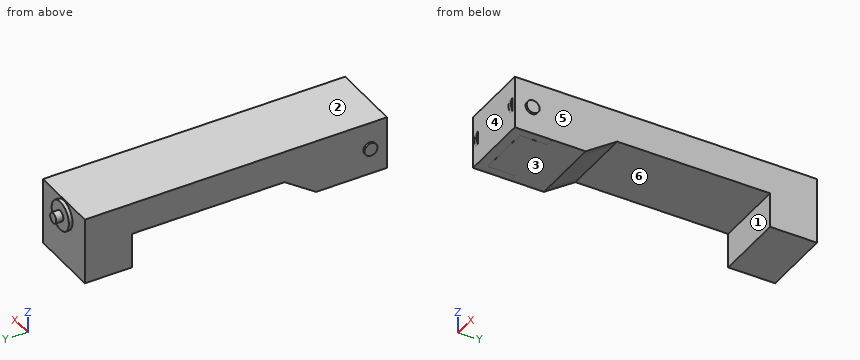
from build123d import *
from OCP.BRepFilletAPI import BRepFilletAPI_MakeChamfer

# Parameters (mm, degrees)
SKETCH1_W            = 41
SKETCH1_H            = 40.2
BOSS_EXTRUDE1_DEPTH  = 61.1
SKETCH2_R            = 14
BOSS_EXTRUDE2_DEPTH  = 3
SKETCH3_R            = 4.9
BOSS_EXTRUDE3_DEPTH  = 4.8
CHAMFER1_SIZE        = 7.5
CHAMFER1_SIZE2       = 5.1
MIRROR5_START        = -20.5
MIRROR5_DEPTH        = 41
BOSS_EXTRUDE4_DEPTH  = 1.5
BOSS_EXTRUDE5_DEPTH  = 4.7625
SKETCH7_W            = 35.6
SKETCH7_H            = 50.6
BOSS_EXTRUDE6_DEPTH  = 35.5
SKETCH9_W            = 29.5
SKETCH9_H            = 35
BOSS_EXTRUDE7_DEPTH  = 39.8
SKETCH10_R           = 11
BOSS_EXTRUDE8_DEPTH  = 2.75
SKETCH11_R           = 3.9
BOSS_EXTRUDE9_DEPTH  = 5.35
SKETCH12_W           = 50.6
SKETCH12_H           = 35.5
BOSS_EXTRUDE10_DEPTH = 8.9625
SKETCH13_W           = 50.6
SKETCH13_H           = 35.5
BOSS_EXTRUDE11_DEPTH = 8.9625
SKETCH14_W           = 53.520973266
SKETCH14_H           = 24
BOSS_EXTRUDE12_DEPTH = 131.85
SKETCH15_W           = 53.525
SKETCH15_H           = 28.80973019
BOSS_EXTRUDE13_DEPTH = 10
SKETCH16_W           = 44
SKETCH16_H           = 7.5
BOSS_EXTRUDE14_DEPTH = 10
SKETCH17_W           = 53.525
SKETCH17_H           = 40.184191337
BOSS_EXTRUDE15_DEPTH = 44


# Read off the part's stored shape, not the designer's step: Mirror5
with BuildPart() as part:
    # Sketch1 → Boss-Extrude1 (new body)
    with BuildSketch(Plane(origin=(0, -13, 0), x_dir=(-1, 0, 0), z_dir=(0, 1, 0))):
        Rectangle(SKETCH1_W, SKETCH1_H)
    extrude(amount=BOSS_EXTRUDE1_DEPTH)

    # Sketch2 → Boss-Extrude2 (add)
    with BuildSketch(Plane.ZY.offset(20.5)):
        with Locations(Location((0, 0, 0), (0, 0, 248.213210702))):
            Circle(SKETCH2_R)
    boss_extrude2 = extrude(amount=BOSS_EXTRUDE2_DEPTH)

    # Sketch3 → Boss-Extrude3 (add)
    with BuildSketch(Plane.ZY.offset(23.5)):
        Circle(SKETCH3_R)
    boss_extrude3 = extrude(amount=BOSS_EXTRUDE3_DEPTH)

    # Chamfer1: one chamfer whose edges measure the first distance from different faces: ONE call of the kernel's chamfer builder (chamfer() names one face for all edges)
    chamfer1_edges_1 = [part.edges().sort_by_distance(p)[0] for p in [
        (0, 48.1, -20.1),
    ]]
    chamfer1_side_1 = [part.faces().sort_by_distance(p)[0] for p in [
        (0, 17.55, -20.1),
    ]]
    chamfer1_edges_2 = [part.edges().sort_by_distance(p)[0] for p in [
        (0, 48.1, 20.1),
    ]]
    chamfer1_side_2 = [part.faces().sort_by_distance(p)[0] for p in [
        (0, 17.55, 20.1),
    ]]
    chamfer1 = BRepFilletAPI_MakeChamfer(part.part.solid().wrapped)
    for e in chamfer1_edges_1:
        chamfer1.Add(CHAMFER1_SIZE, CHAMFER1_SIZE2, e.wrapped, chamfer1_side_1[0].wrapped)  # the first distance lies on this face
    for e in chamfer1_edges_2:
        chamfer1.Add(CHAMFER1_SIZE, CHAMFER1_SIZE2, e.wrapped, chamfer1_side_2[0].wrapped)  # the first distance lies on this face
    add(Compound.cast(chamfer1.Shape()), mode=Mode.REPLACE)

    # Mirror5 outline → Mirror5 (cut)
    with BuildSketch(Plane.YZ.offset(MIRROR5_START)):
        Polygon((-13, 20.1), (-13, 15), (-5.5, 20.1), align=None)
        Polygon((-5.5, -20.1), (-13, -15), (-13, -20.1), align=None)
    extrude(amount=MIRROR5_DEPTH, mode=Mode.SUBTRACT)

    # Sketch4 → Boss-Extrude4 (add)
    with BuildSketch(Plane.ZY.offset(20.5)):
        Polygon((-20.1, 15.2), (20.1, 15.2), (20.1, 40.6), (15, 48.1), (-15, 48.1), (-20.1, 40.6), align=None)
    boss_extrude4 = extrude(amount=BOSS_EXTRUDE4_DEPTH)

    # Mirror1: Boss-Extrude2, Boss-Extrude3, Boss-Extrude4 across plane
    add(boss_extrude2.mirror(Plane(origin=(0, 0, 0), x_dir=(0, 0, 1), z_dir=(1, 0, 0))))
    add(boss_extrude3.mirror(Plane(origin=(0, 0, 0), x_dir=(0, 0, 1), z_dir=(1, 0, 0))))
    add(boss_extrude4.mirror(Plane(origin=(0, 0, 0), x_dir=(0, 0, 1), z_dir=(1, 0, 0))))

    # Sketch6 → Boss-Extrude5 (add)
    with BuildSketch(Plane(origin=(22, 0, 0), x_dir=(0, 0, -1), z_dir=(1, 0, 0))):
        Polygon((20.1, 15.2), (20.1, 40.6), (3.9, 64.423529412), (3.9, 215.2), (-20.1, 215.2), (-20.1, 25.2), (4.9, 15.2), align=None)
    boss_extrude5 = extrude(amount=BOSS_EXTRUDE5_DEPTH)

    # Mirror2: Boss-Extrude5 across plane
    add(boss_extrude5.mirror(Plane(origin=(0, 0, 0), x_dir=(0, 0, 1), z_dir=(1, 0, 0))))



with BuildPart() as body_2:
    # Sketch7 → Boss-Extrude6 (new body)
    with BuildSketch(Plane(origin=(0, 215.45, 0), x_dir=(-1, 0, 0), z_dir=(0, 1, 0))):
        with Locations((0, -5.2)):
            Rectangle(SKETCH7_W, SKETCH7_H)
    extrude(amount=-BOSS_EXTRUDE6_DEPTH)


with BuildPart() as part_1:
    add(part.part)

    add(body_2.part)  # Boss-Extrude7 merges body 2
    # Sketch9 → Boss-Extrude7 (add)
    with BuildSketch(Plane.ZY.offset(-22)):
        with Locations((5.35, 197.7)):
            Rectangle(SKETCH9_W, SKETCH9_H)
    boss_extrude7 = extrude(amount=BOSS_EXTRUDE7_DEPTH)

    # Mirror3: Boss-Extrude7 across plane
    add(boss_extrude7.mirror(Plane(origin=(0, 0, 0), x_dir=(0, 0, 1), z_dir=(1, 0, 0))))

    # Sketch10 → Boss-Extrude8 (add)
    with BuildSketch(Plane(origin=(0, 215.45, 0), x_dir=(-1, 0, 0), z_dir=(0, 1, 0))):
        with Locations(Location((0, 8.1, 0), (0, 0, 270))):
            Circle(SKETCH10_R)
    extrude(amount=BOSS_EXTRUDE8_DEPTH)

    # Sketch11 → Boss-Extrude9 (add)
    with BuildSketch(Plane(origin=(0, 218.2, 0), x_dir=(-1, 0, 0), z_dir=(0, 1, 0))):
        with Locations(Location((0, 8.1, 0), (0, 0, 90))):
            Circle(SKETCH11_R)
    extrude(amount=BOSS_EXTRUDE9_DEPTH)

    # Sketch12 → Boss-Extrude10 (add)
    with BuildSketch(Plane(origin=(17.8, 0, 0), x_dir=(0, 0, -1), z_dir=(1, 0, 0))):
        with Locations((5.2, 197.7)):
            Rectangle(SKETCH12_W, SKETCH12_H)
    extrude(amount=BOSS_EXTRUDE10_DEPTH)

    # Sketch13 → Boss-Extrude11 (add)
    with BuildSketch(Plane.ZY.offset(17.8)):
        with Locations((-5.2, 197.7)):
            Rectangle(SKETCH13_W, SKETCH13_H)
    extrude(amount=BOSS_EXTRUDE11_DEPTH)

    # Sketch14 → Boss-Extrude12 (add)
    with BuildSketch(Plane.XZ.offset(-179.95)):
        with Locations((-0.002013367, 8.1)):
            Rectangle(SKETCH14_W, SKETCH14_H)
    extrude(amount=BOSS_EXTRUDE12_DEPTH)

    # Sketch15 → Boss-Extrude13 (add)
    with BuildSketch(Plane(origin=(0, 22.183698031, -32.623085339), x_dir=(-1, 0, 0), z_dir=(0, 0.562310021407278, -0.826926502069529))):
        with Locations((0, 36.675649649)):
            Rectangle(SKETCH15_W, SKETCH15_H)
    extrude(amount=-BOSS_EXTRUDE13_DEPTH)

    # Sketch16 → Boss-Extrude14 (add)
    with BuildSketch(Plane.XY.offset(20.1)):
        with Locations((0, 44.35)):
            Rectangle(SKETCH16_W, SKETCH16_H)
    extrude(amount=-BOSS_EXTRUDE14_DEPTH)

    # Sketch17 → Boss-Extrude15 (add)
    with BuildSketch(Plane.XZ.offset(13)):
        with Locations((0, 0.007904332)):
            Rectangle(SKETCH17_W, SKETCH17_H)
    extrude(amount=-BOSS_EXTRUDE15_DEPTH)


solid = part_1.part
Check sheet for the modelled part. Datum: model origin and axes. Units: mm. Face numbers are marked on the shaded views. A direction names the side the tool comes from. Coordinates: 2 decimals unless noted, no trailing zeros. Loops run counter-clockwise (first coordinate to the right, second up) from the corner with the lowest first, then second, coordinate; pieces in that order, holes last. Notation, with made-up numbers: (82.25, -26) -> (127.25, -26) arc R17 cw to (127.25, -16) -> close; hole circle Ø8 at (39.5, 35.5). An arc over 180 degrees is marked (long way). Answer in a Markdown table with one row per item.
1. Material ranges on line 1 along X through (y, z) = (19, 1); line 2 along Y through (x, z) = (-6.5, 1.5); line 3 along Z through (x, y) = (3, 2.5), recorded low to high. Write a range as [from, to].
Check values:
| item | result |
|---|---|
| line 1 | x = [-26.76, 26.76] |
| line 2 | y = [-13, 218.2] |
| line 3 | z = [-20.1, 20.1] |
2. Access from +Z, -Z, +X, -X, +Y, -Y to the whole of each face (thin tool, end or side, straight path). Record for the marked faces 1, 2 and 3.
Check values:
| item | result |
|---|---|
| face 1 | -Z, +X, -X |
| face 2 | +Z, +X, -X, +Y, -Y |
| face 3 | -Z, +X, -X, -Y |
3. Sectioned sample at D-D, the plane z = 8.1. Record the boundary of the cut face in (x, y), then the cut area to 3 significant figures.
Check values:
| item | result |
|---|---|
| outline | (-26.76, -13) -> (26.76, -13) -> (26.76, 215.45) -> (11, 215.45) -> (11, 218.2) -> (3.9, 218.2) -> (3.9, 223.55) -> (-3.9, 223.55) -> (-3.9, 218.2) -> (-11, 218.2) -> (-11, 215.45) -> (-26.76, 215.45) -> close |
| area | 12,300 mm2 |
4. Go/stop test with flat-tipped pins: pin 1 (1 mm diameter, centred on x = 15, z = 3, fed in from +Y); pin 2 (2 mm diameter, centred on x = 6, z = 6, fed in from -Y); pin 3 (22.5 mm diameter, centred on x = -3.5, y = 8, fed in from -Z); pin 4 (1 mm diameter, centred on y = 178, z = -11, fed in from -X). Record where each tip stops, or that it passes through.
Check values:
| item | result |
|---|---|
| pin 1 | stops at y = 215.45 |
| pin 2 | stops at y = -13 |
| pin 3 | stops at z = -20.1 |
| pin 4 | passes through |
5. Sectioned sample at B-B, the plane z = -11.5. Record the boundary of the cut face in (x, y), then the cut area to 3 significant figures.
Check values:
| item | result |
|---|---|
| outline | (-26.76, -13) -> (26.76, -13) -> (26.76, 53.25) -> (-26.76, 53.25) -> close; (-26.76, 179.95) -> (26.76, 179.95) -> (26.76, 215.45) -> (-26.76, 215.45) -> close |
| area | 5,450 mm2 |
6. Release check for a two-part mould opening along X. For the marked faces 4, 5 and 6 record: released by +X, released by -X, zero draft, split by the parting line, or undercut.
Check values:
| item | result |
|---|---|
| face 4 | undercut |
| face 5 | released by +X |
| face 6 | zero draft |
